Part print with two shaded views. Sizes in mm from the minimum x, y, z corner. A direction names the side the tool comes from. Coordinates: 2 decimals unless noted, no trailing zeros. Loops run counter-clockwise (first coordinate to the right, second up) from the corner with the lowest first, then second, coordinate; pieces in that order, holes last.
Item 1: 3-axis set-ups, long thin cutter, end or side, ignore diameter. For the marked faces 4 and 5: which of +Z, -Z, +X, -X, +Y, -Y reach the whole face in a straight line?
Item 2: Cut at B-B (z = 25.4). List the corners of the cut face in (x, y) (1 decimal), and give its area (3 significant figures).
Item 3: Drill centre lines: line 1 along Z through (x, y) = (19.05, 11.5) (1 decimal); line 2 along Z through (x, y) = (4, 12.7); line 3 along Y through (x, z) = (30.75, 25.4). Where is each one in solid material? Low to high.
Item 4: Cut at C-C (x = 19.05). List the corners of the cut face in (y, z) (1 decimal).
Item 5: Cut at D-D (z = 45). List the corners of the cut face in (x, y).
Item 6: Cut at A-A (y = 12.7). Count the separate pieces of the cut face and the enclosed holes in it, and give its area (3 significant figures).
Item 7: Mould opens along X. For the marked faces 1, 2 and 3 say: released by +X, released by -X, zero draft, split by the parting line, or undercut.
Item 8: Flat gauge pins, fed straight in: pin 1 (7.5 mm diameter, centred on x = 65, y = 10, fed in from +Z) (1 decimal); pin 2 (5.5 mm diameter, centred on y = 12.7, z = 52.39, fed in from +X). Where does each tip first touch, or does it go through?
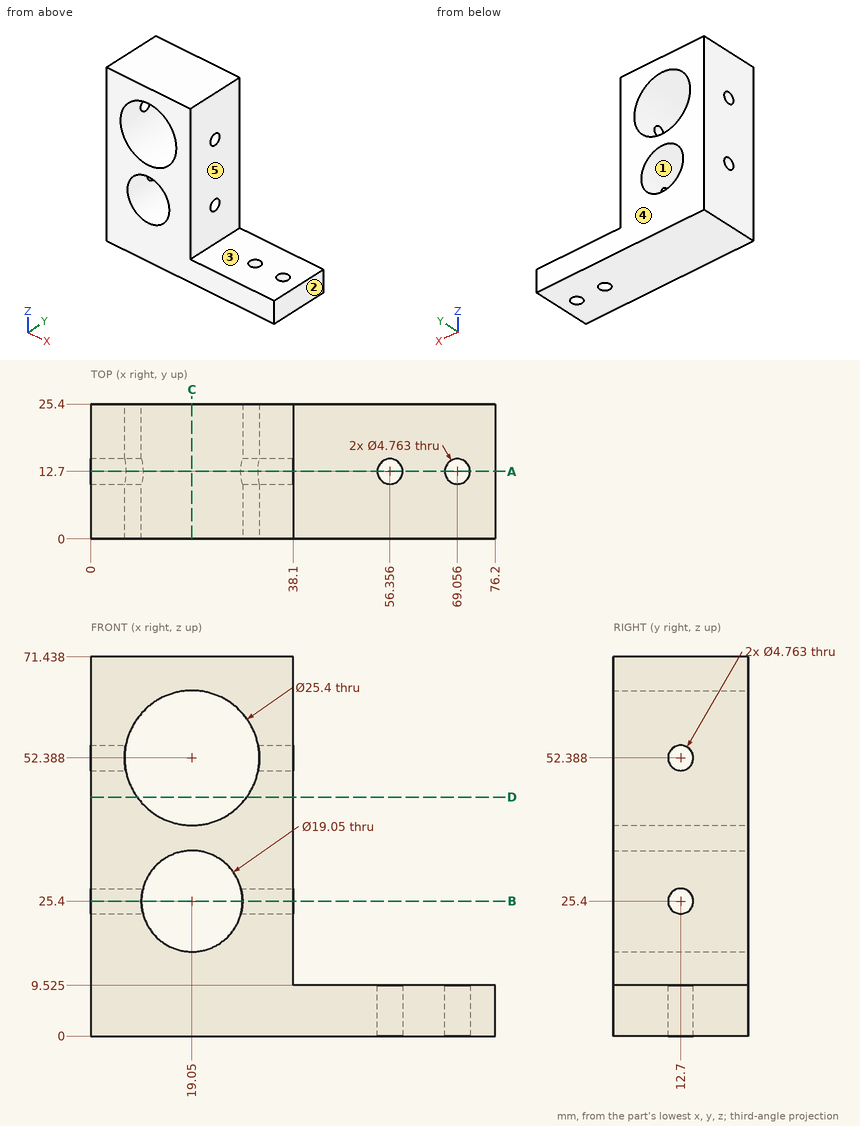
Filled sheet:
1. face 4: +Z, -Z, +X, -X, +Y
1. face 5: +Z, +X, +Y, -Y
2. outline: (0, 0) - (9.5, 0) - (9.5, 10.3) - (0, 10.3) - close; (0, 15.1) - (9.5, 15.1) - (9.5, 25.4) - (0, 25.4) - close; (28.6, 0) - (38.1, 0) - (38.1, 10.3) - (28.6, 10.3) - close; (28.6, 15.1) - (38.1, 15.1) - (38.1, 25.4) - (28.6, 25.4) - close
2. area: 393 mm2
3. line 1: z = 0 to 15.9, 34.9 to 39.7, 65.1 to 71.4
3. line 2: z = 0 to 23.02, 27.78 to 50.01, 54.77 to 71.44
3. line 3: y = 0 to 10.32, 15.08 to 25.4
4. outline: (0, 0) - (25.4, 0) - (25.4, 15.9) - (0, 15.9) - close; (0, 34.9) - (25.4, 34.9) - (25.4, 39.7) - (0, 39.7) - close; (0, 65.1) - (25.4, 65.1) - (25.4, 71.4) - (0, 71.4) - close
5. outline: (0, 0) - (8.72, 0) - (8.72, 25.4) - (0, 25.4) - close; (29.38, 0) - (38.1, 0) - (38.1, 25.4) - (29.38, 25.4) - close
6. separate pieces: 5
6. enclosed holes: 0
6. area: 2,050 mm2
7. face 1: undercut
7. face 2: released by +X
7. face 3: zero draft
8. pin 1: stops at z = 9.5
8. pin 2: stops at x = 38.1
